Part model, mm, in its own coordinate system. Round coordinates to 2 decimals unless told otherwise and drop trailing zeros. Loops run counter-clockwise (first coordinate to the right, second up) from the corner with the lowest first, then second, coordinate; pieces in that order, holes last. Notation, with made-up numbers: M 83,24 L 109,24 A14 cw 109,29 Z; hole C 74.5,66.5 d10. An arc over 180 degrees is marked long. Write each question's results on one line, items separated by ' | '.
from build123d import *

# Parameters (mm, degrees)
SKETCH3_R           = 14.2748
SKETCH3_R_2         = 7.9375
SKETCH3_R_3         = 2.4892
SKETCH3_R_4         = 3.175
BOSS_EXTRUDE1_DEPTH = 6.35
CHAMFER1_SIZE       = 2.54


with BuildPart() as part:
    # Sketch3 → Boss-Extrude1 (new body)
    with BuildSketch(Plane(origin=(0, 0, 0), x_dir=(1, 0, 0), z_dir=(0, 1, 0))):
        with BuildLine():
            Line((-249.735512242, 346.01236887), (-239.395, 346.01236887))
            ThreePointArc((-239.395, 346.01236887), (-237.14993597, 345.0824329), (-236.22, 342.83736887))
            Line((-236.22, 342.83736887), (-236.22, 317.5))
            ThreePointArc((-236.22, 317.5), (-231.880567419, 303.300968343), (-220.345, 293.953569803))
            Line((-220.345, 293.953569803), (-220.345, 285.75))
            ThreePointArc((-220.345, 285.75), (-210.82, 276.225), (-201.295, 285.75))
            Line((-201.295, 285.75), (-201.295, 293.953569803))
            ThreePointArc((-201.295, 293.953569803), (-189.759432581, 303.300968343), (-185.42, 317.5))
            Line((-185.42, 317.5), (-185.42, 548.034576396))
            ThreePointArc((-185.42, 548.034576396), (-210.82, 573.434576396), (-236.22, 548.034576396))
            Line((-236.22, 548.034576396), (-236.22, 397.808393354))
            ThreePointArc((-236.22, 397.808393354), (-237.14993597, 395.563329324), (-239.395, 394.633393354))
            Line((-239.395, 394.633393354), (-249.735512242, 394.633393354))
            ThreePointArc((-249.735512242, 394.633393354), (-251.980576272, 393.703457384), (-252.910512242, 391.458393354))
            Line((-252.910512242, 391.458393354), (-252.910512242, 349.18736887))
            ThreePointArc((-252.910512242, 349.18736887), (-251.980576272, 346.942304839), (-249.735512242, 346.01236887))
        make_face()
        with Locations((-210.82, 548.034576396)):
            Circle(SKETCH3_R, mode=Mode.SUBTRACT)
        with Locations((-210.82, 438.027176396)):
            Circle(SKETCH3_R, mode=Mode.SUBTRACT)
        with Locations((-210.82, 317.5)):
            Circle(SKETCH3_R, mode=Mode.SUBTRACT)
        with Locations((-228.6, 370.322881112)):
            Circle(SKETCH3_R_2, mode=Mode.SUBTRACT)
        with Locations((-246.560512242, 388.283393354)):
            Circle(SKETCH3_R_3, mode=Mode.SUBTRACT)
        with Locations((-210.639487758, 352.36236887)):
            Circle(SKETCH3_R_3, mode=Mode.SUBTRACT)
        with Locations((-210.82, 285.75)):
            Circle(SKETCH3_R_4, mode=Mode.SUBTRACT)
        with Locations((-210.82, 493.030876396)):
            Circle(SKETCH3_R_4, mode=Mode.SUBTRACT)
        with Locations((-195.58, 370.322881112)):
            Circle(SKETCH3_R_4, mode=Mode.SUBTRACT)
    extrude(amount=BOSS_EXTRUDE1_DEPTH)

    # Chamfer1
    chamfer1_edges = [part.edges().sort_by_distance(p)[0] for p in [
        (-213.995, 6.35, -493.030876396),
        (-213.995, 0, -493.030876396),
    ]]
    chamfer(chamfer1_edges, length=CHAMFER1_SIZE)


solid = part.part
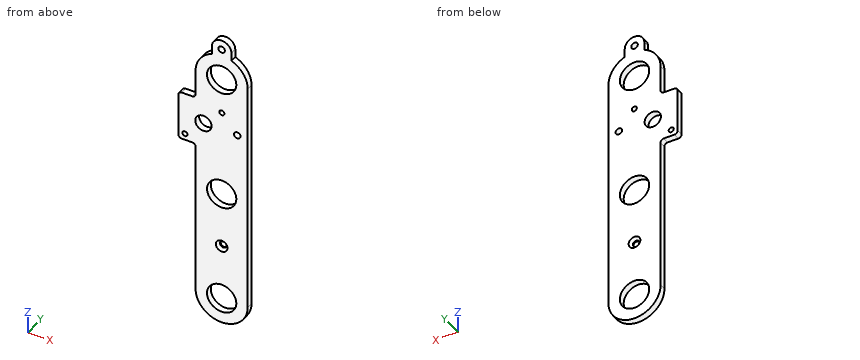
Item 1: Drop flat-ended pins along their axis: P1, Ø3, axis at x = -201, y = 1.5, coming from the +Z side; P2, Ø4.5, axis at x = -246.56, z = -388.28, coming from the -Y side; P3, Ø1.9, axis at x = -247, y = 4.5, coming from the +Z side; P4, Ø10, axis at x = -210.82, z = -493.03, coming from the +Y side. Give the stop position or say it passes through.
Filled sheet:
P1: z = -281.11 | P2: through | P3: z = -346.01 | P4: y = 5.64
Item 2: Band-saw the part on C-C on z = -443.5. Give the cut face in (x, y), and give its area (3 significant figures).
Filled sheet:
outline: M -236.22,0 L -224,0 L -224,6.35 L -236.22,6.35 Z; M -197.64,0 L -185.42,0 L -185.42,6.35 L -197.64,6.35 Z | area: 155 mm^2
Item 3: Band-saw the part on B-B on x = -228.6. Give the cut face in (y, z), and give its area (3 significant figures).
Filled sheet:
outline: M 0,-566.17 L 6.35,-566.17 L 6.35,-378.26 L 0,-378.26 Z; M 0,-362.39 L 6.35,-362.39 L 6.35,-299.36 L 0,-299.36 Z | area: 1,590 mm^2
Item 4: Band-saw the part on D-D on z = -299.5. Give the cut face in (x, y).
Filled sheet:
outline: M -228.74,0 L -192.9,0 L -192.9,6.35 L -228.74,6.35 Z
Item 5: Wall check: L1, parallel to X at y = 4, z = -285.75 (3 decimals); L2, parallel to Z at x = -250, y = 4.5; L3, parallel to Z at x = -228.6, y = 4.5. Give the ranges that are in metal, low to high.
Filled sheet:
L1: -220.345 to -213.995, -207.645 to -201.295 | L2: -394.62 to -346.02 | L3: -566.17 to -378.26, -362.39 to -299.36
Item 6: Band-saw the part on A-A on y = 5.25. Count the separate pieces of the cut face and the enclosed holes in it, and give its area (3 significant figures).
Filled sheet:
separate pieces: 1 | enclosed holes: 9 | area: 12,500 mm^2
